The listing builds one solid part. Answer for the finished solid, in the listing's coordinates (mm). A direction names the side the tool comes from. Coordinates: 2 decimals unless noted, no trailing zeros. Loops run counter-clockwise (first coordinate to the right, second up) from the corner with the lowest first, then second, coordinate; pieces in that order, holes last. Notation, with made-up numbers: (82.25, -0.5) - (128.25, -0.5) arc R17 ccw to (128.25, 21.5) - close; hole circle Ø6 at (-22.5, 46.25). An arc over 180 degrees is marked (long way). Write each question's results on one line, items separated by ' | '. Start each with the question number.
(1) For faces 5 (the flat face through (0, 64, 3.464)), 6 (the cylindrical face through (3, 61, 0)), determine the directions among +Z, -Z, +X, -X, +Y, -Y from which every point of the face is accessible in a straight line to the end or side of a thin tool.
(2) Given pin 1 Ø1 at (x, z) = (-0.5, 0.5) entering from +Y; pin 2 Ø3 at (x, z) = (-2, 2.5) entering from +Y; pin 3 Ø1 at (y, z) = (63, 1.5) entering from +X, each flat-ended and moving along its own axis, determine where each tip first touches the part or whether it passes through.
(3) Determine the mould class of faces 1 (the flat face through (2, 135, -1)), 2 (the flat face through (-3.014, 64.267, 1.708)), 3 (the flat face through (3.014, 64.267, -1.708)), 4 (the cylindrical face through (2, 131, 0)) for opening direction Z: released by +Z, released by -Z, zero draft, split by the parting line, or undercut.
(4) Find section A-A on y = 37. Determine the outline of the cut face in (x, z).
(5) Consider line 1 (Z direction, x = -0.75, y = 94); line 2 (Z direction, x = 0.5, y = 46); line 3 (X direction, y = 105, z = -2.25). Determine where each line is inside the solid, lowest interval first. Write a range as from..to.
from build123d import *

# Parameters (mm, degrees)
CROQUIS1_R              = 4
CROQUIS1_R_2            = 3
SALIENTE_EXTRUIR1_DEPTH = 125
CORTAR_EXTRUIR1_DEPTH   = 136.11846654
REDONDEO1_R             = 4
CROQUIS15_R             = 3.25
CROQUIS15_R_2           = 3.15
CORTAR_EXTRUIR2_DEPTH   = 0.05
CROQUIS17_R             = 0.5
CORTAR_EXTRUIR3_DEPTH   = 1


with BuildPart() as part:
    # Croquis1 → Saliente-Extruir1 (new body)
    with BuildSketch(Plane(origin=(0, 0, 0), x_dir=(1, 0, 0), z_dir=(0, 1, 0))):
        with Locations(Location((0, 0, 0), (0, 0, 270))):
            Circle(CROQUIS1_R)
        with Locations(Location((0, 0, 0), (0, 0, 270))):
            Circle(CROQUIS1_R_2, mode=Mode.SUBTRACT)
    extrude(amount=SALIENTE_EXTRUIR1_DEPTH)

    # Croquis13 → Revolución1 (revolve)
    with BuildSketch(Plane.XY, mode=Mode.PRIVATE) as revoluci_n1_sk:
        with BuildLine():
            Line((-4, 125), (-3, 135))
            Line((-3, 135), (-2, 135))
            Line((-2, 135), (-2, 127.267949192))
            ThreePointArc((-2, 127.267949192), (-2.068148347, 126.750311102), (-2.267949192, 126.267949192))
            Line((-2.267949192, 126.267949192), (-3, 125))
            Line((-3, 125), (-4, 125))
        make_face()
    revolve(revoluci_n1_sk.sketch.rotate(Axis((0, 125, 0), (0, 1, 0)), 270), axis=Axis((0, 125, 0), (0, 1, 0)))

    # Croquis14 → Cortar-Extruir1 (cut, through all)
    with BuildSketch(Plane.XZ):
        with BuildLine():
            Line((2, -3.464101615), (-2, -3.464101615))
            ThreePointArc((-2, -3.464101615), (0, -4), (2, -3.464101615))
        make_face()
        with BuildLine():
            Line((4, 0), (2, -3.464101615))
            ThreePointArc((2, -3.464101615), (3.464101615, -2), (4, 0))
        make_face()
        with BuildLine():
            ThreePointArc((4, 0), (3.464101615, 2), (2, 3.464101615))
            Line((2, 3.464101615), (4, 0))
        make_face()
        with BuildLine():
            ThreePointArc((2, 3.464101615), (0, 4), (-2, 3.464101615))
            Line((-2, 3.464101615), (2, 3.464101615))
        make_face()
        with BuildLine():
            ThreePointArc((-2, 3.464101615), (-3.464101615, 2), (-4, 0))
            Line((-4, 0), (-2, 3.464101615))
        make_face()
        with BuildLine():
            Line((-2, -3.464101615), (-4, 0))
            ThreePointArc((-4, 0), (-3.464101615, -2), (-2, -3.464101615))
        make_face()
    extrude(amount=-CORTAR_EXTRUIR1_DEPTH, mode=Mode.SUBTRACT)

    # Redondeo1
    redondeo1_edges = [part.edges().sort_by_distance(p)[0] for p in [
        (-3, 125, 0),
    ]]
    fillet(redondeo1_edges, radius=REDONDEO1_R)

    # Croquis15 → Cortar-Extruir2 (cut)
    with BuildSketch(Plane.XZ):
        with Locations(Location((0, 0, 0), (0, 0, 270))):
            Circle(CROQUIS15_R)
        with Locations(Location((0, 0, 0), (0, 0, 270))):
            Circle(CROQUIS15_R_2, mode=Mode.SUBTRACT)
    extrude(amount=-CORTAR_EXTRUIR2_DEPTH, mode=Mode.SUBTRACT)

    # Croquis17 → Cortar-Extruir3 (cut)
    with BuildSketch(Plane.XY.offset(3.464101615)):
        with Locations((0, 60)):
            Circle(CROQUIS17_R)
    extrude(amount=-CORTAR_EXTRUIR3_DEPTH, mode=Mode.SUBTRACT)


solid = part.part
Values:
1) face 5: +Z, +X, -X, +Y, -Y | face 6: -Y
2) pin 1: passes through | pin 2: stops at y = 135 | pin 3: stops at x = 3.42
3) face 1: zero draft | face 2: released by +Z | face 3: released by -Z | face 4: undercut
4) outline: (-4, 0) - (-2, -3.46) - (2, -3.46) - (4, 0) - (2, 3.46) - (-2, 3.46) - close; hole circle Ø6 at (0, 0)
5) line 1: z = -3.46..-2.9, 2.9..3.46 | line 2: z = -3.46..-2.96, 2.96..3.46 | line 3: x = -2.7..-1.98, 1.98..2.7
